Autodesk Inventor part; units mm, degrees
ref_plane "YZ Plane" through (0, 0, 0) normal (1, 0, 0) x (0, 1, 0)
ref_plane "XZ Plane" through (0, 0, 0) normal (0, 1, 0) x (-1, 0, 0)
ref_plane "XY Plane" through (0, 0, 0) normal (0, 0, 1) x (1, 0, 0)
sketch "Эскиз1" plane through (0, 0, 0) normal (0, 1, 0) x (-1, 0, 0)
  line L0 (0, 0) -> (12, 0)
  line L1 (12, 0) -> (12, -28)
  line L2 (12, -28) -> (0, -28)
  line L3 (0, -28) -> (0, 0)
  circle A0 centre (6, -12) radius 0.65
  circle A1 centre (6, -17) radius 0.65
  circle A2 centre (6, -22) radius 0.65
  line L4 (6, -12) -> (6, -17) construction
  line L5 (6, -17) -> (6, -22) construction
  line L6 (6, -6) -> (6, 0) construction
  line L7 (6, -12) -> (12, -12) construction
  circle A3 centre (6, -17) radius 1.15
  circle A4 centre (6, -12) radius 1.15
  circle A5 centre (6, -22) radius 1.15
  circle A6 centre (6, -6) radius 2.25
  line L8 (6, -12) -> (6, -6) construction
  line L9 (6, -22) -> (6, -28) construction
  point P0 (12, -14)
  dimension "d1" = 5
  dimension "d4" = 6
  dimension "d5" = 1.3
  dimension "d6" = 0.5
  dimension "d30" = 6
  dimension "d31" = 4.5
extrude "Выдавливание1" add sketch "Эскиз1" against normal blind 2 contours L0 L1 L2 L3 | A0 | A1 | A2 | A3 | A4 | A5 | A6
extrude "Выдавливание2" add sketch "Эскиз1" along normal blind 0.5 contours A4
extrude "Выдавливание4" add sketch "Эскиз1" along normal blind 1.6 contours A3
extrude "Выдавливание5" add sketch "Эскиз1" along normal blind 3.2 contours A5
sketch "Эскиз2" plane through (-6, 1.6, -17) normal (0, 1, 0) x (1, 0, 0)
  circle A0 centre (0, 0) radius 0.65
  point P0 (6, -17)
extrude "Выдавливание3" cut sketch "Эскиз2" against normal through all
extrude "Выдавливание7" cut sketch "Эскиз1" against normal through all contours A6
sketch "Эскиз7" plane through (0, -2, 0) normal (0, -1, 0) x (1, 0, 0)
  circle A0 centre (-6, -6) radius 2.25
  line L0 (-1, -10) -> (-11, -10)
  line L1 (-11, -10) -> (-11, -2)
  line L2 (-11, -2) -> (-1, -2)
  line L3 (-1, -2) -> (-1, -10)
  line L4 (-1, -10) -> (-11, -2) construction
  line L5 (-11, -10) -> (-1, -2) construction
  point P0 (0, 0)
  dimension "d34" = 10
  dimension "d35" = 8
extrude "Выдавливание8" cut sketch "Эскиз7" against normal blind 1.3
sketch "Эскиз5" plane through (0, 0, 0) normal (0, 1, 0) x (1, 0, 0)
  circle A0 centre (-1.1, 1.1) radius 0.7
  line L0 (0, 0) -> (0, 28)
  line L1 (0, 0) -> (-12, 0) construction
  line L2 (-6, 0) -> (-6, 28) construction
  line L3 (-12, 28) -> (0, 28) construction
  line L4 (-12, 0) -> (-12, 28) construction
  line L5 (-12, 14) -> (0, 14) construction
  circle A1 centre (-10.9, 1.1) radius 0.7
  circle A2 centre (-1.1, 26.9) radius 0.7
  circle A3 centre (-10.9, 26.9) radius 0.7
  dimension "d17" = 1.1
  dimension "d18" = 1.4
  dimension "d19" = 1.1
extrude "Выдавливание6" add sketch "Эскиз5" along normal blind 0.2
sketch "Эскиз6" plane through (-10.9, 0.2, -1.1) normal (0, 1, 0) x (1, 0, 0)
  circle A0 centre (0, 0) radius 0.7
  circle A1 centre (9.8, 0) radius 0.7
  circle A2 centre (9.8, 25.8) radius 0.7
  circle A3 centre (0, 25.8) radius 0.7
  point P0 (10.9, -1.1)
hole "Отверстие1" at (-10.9, 0.2, -1.1) at (-1.1, 0.2, -1.1) at (-10.9, 0.2, -26.9) at (-1.1, 0.2, -26.9) direction (0, -1, 0) diameter 1 end through all
fillet "Сопряжение1" radius 1 4 edges at (0, -1, 0) (-12, -1, 0) (0, -1, -28) (-12, -1, -28)
equation "\"d19\" = d17"
properties part number "Основание сервы"
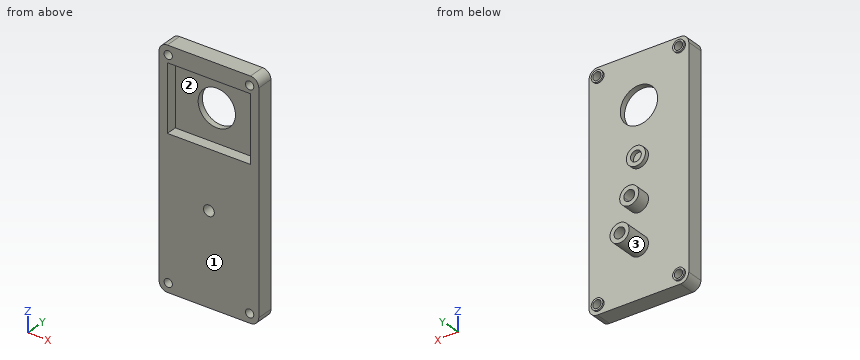
Input: part model. Units: mm. Frame: model coordinates. Face numbers are marked on the shaded views. Round coordinates to 2 decimals unless told otherwise and drop trailing zeros. Loops run counter-clockwise (first coordinate to the right, second up) from the corner with the lowest first, then second, coordinate; pieces in that order, holes last. Notation, with made-up numbers: (77, -26.75) -> (123, -26.75) arc R15 ccw to (123, -6.75) -> close; hole circle Ø7 at (-19, 51). An arc over 180 degrees is marked (long way). One line per item, written item: value.
(1) Section C-C (x = -9.75). Return the cut outline in (y, z), plus the area to 3 significant figures.
Geometry check:
outline: (-2, -28) -> (0, -28) -> (0, 0) -> (-2, 0) -> (-2, -2) -> (-0.7, -2) -> (-0.7, -10) -> (-2, -10) -> close
area: 45.6 mm2
(2) Pin query (flat end, axial travel): pin 1 (1.7 mm diameter, centred on x = -6, z = -17, fed in from +Y); pin 2 (1 mm diameter, centred on y = 1, z = -15, fed in from +X); pin 3 (0.7 mm diameter, centred on x = -5.5, z = -12, fed in from +Y); pin 4 (0.7 mm diameter, centred on x = -6, z = -12, fed in from +Y). Return the tip coordinate at first contact, or that it passes through.
Geometry check:
pin 1: y = 1.6
pin 2: through
pin 3: y = 0.5
pin 4: y = 0
(3) Material intervals for line 1 (X direction, y = -0.3, z = -1.1); line 2 (Z direction, x = -1.1, y = -0.35); line 3 (Z direction, x = -1.1, y = -1.5), sorted ascending. Write a range as [from, to].
Geometry check:
line 1: [-12, -11.4], [-10.4, -1.6], [-0.6, 0]
line 2: [-28, -27.4], [-26.4, -1.6], [-0.6, 0]
line 3: [-28, -27.4], [-26.4, -10], [-2, -1.6], [-0.6, 0]
(4) Mould query, pull axis X, two halves, no side actions, for the marked faces 1, 2 and 3. Classes: pulls with the +X half, pulls with the -X half, needs draft (parallel to the pull), parting line crosses it, or undercut.
Geometry check:
face 1: needs draft
face 2: undercut
face 3: parting line crosses it
(5) Section D-D (x = -6). Give the number of separate pieces and of enclosed holes in the cut face, plus the area to 4 significant figures.
Geometry check:
separate pieces: 3
enclosed holes: 0
area: 45.15 mm2
(6) Section A-A (z = -6). Return the cut outline in (x, y), plus the area to 3 significant figures.
Geometry check:
outline: (-12, -2) -> (-11, -2) -> (-11, -0.7) -> (-8.25, -0.7) -> (-8.25, 0) -> (-12, 0) -> close; (-3.75, -0.7) -> (-1, -0.7) -> (-1, -2) -> (0, -2) -> (0, 0) -> (-3.75, 0) -> close
area: 7.85 mm2
(7) Section B-B (y = -0.3). Return the cut outline in (x, z).
Geometry check:
outline: (-12, -27) arc R1 ccw to (-11, -28) -> (-1, -28) arc R1 ccw to (0, -27) -> (0, -1) arc R1 ccw to (-1, 0) -> (-11, 0) arc R1 ccw to (-12, -1) -> close; hole circle Ø1 at (-10.9, -26.9); hole circle Ø1 at (-10.9, -1.1); hole circle Ø4.5 at (-6, -6); hole circle Ø1.3 at (-6, -17); hole circle Ø1 at (-1.1, -26.9); hole circle Ø1 at (-1.1, -1.1)
